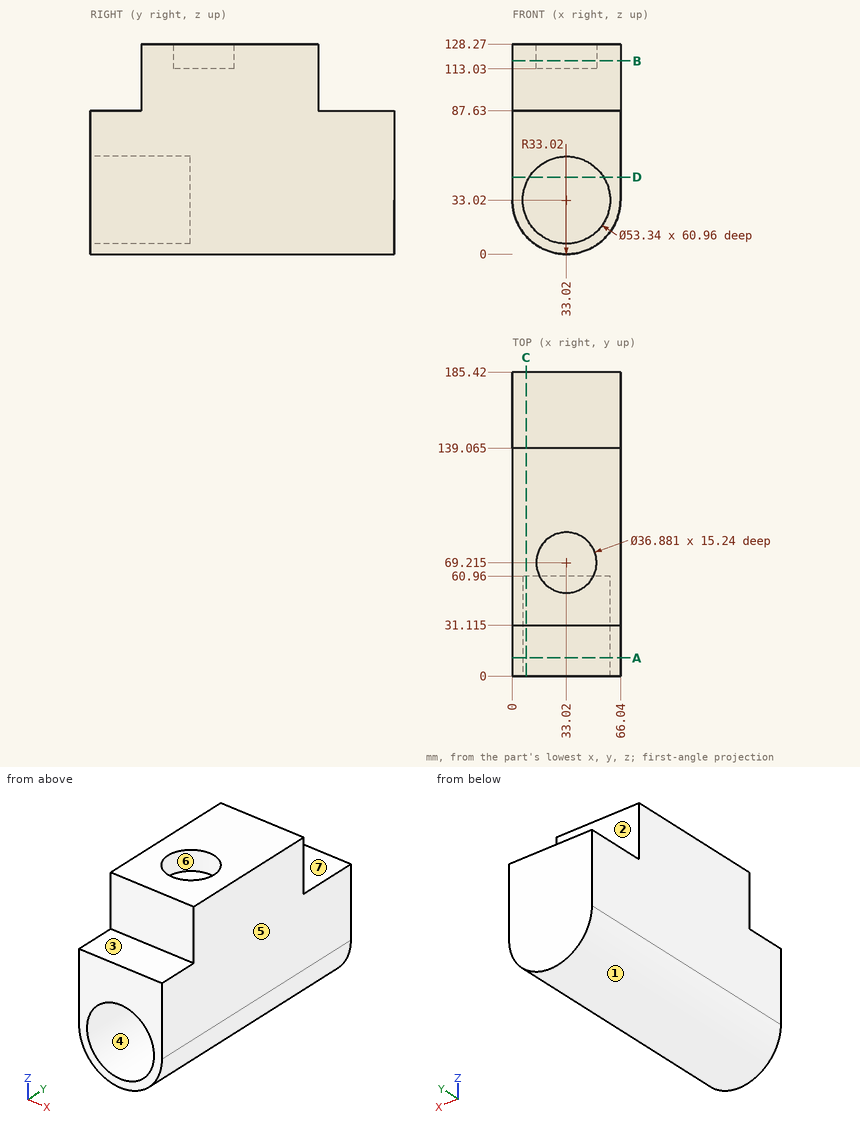
Here's the drawing with two shaded views (mm, measured from the low corner). I have some questions. A direction names the side the tool comes from. Give positions to 0.01 mm unless a question says otherwise; leave off trailing zeros. Loops run counter-clockwise (first coordinate to the right, second up) from the corner with the lowest first, then second, coordinate; pieces in that order, holes last. Notation, with made-up numbers: M 15,52.5 L 61,52.5 A25 ccw 61,86.5 Z; hole C 73,63 d10. An arc over 180 degrees is marked long. One line per item, written item: value.
(1) We'd pull the mould along X, two halves only. Please class the marked faces 4, 5, 6 and 7: released by +X, released by -X, zero draft, split by the parting line, or undercut.
Returned:
face 4: undercut
face 5: released by +X
face 6: undercut
face 7: zero draft
(2) Will these pins go through, and if not, where does the flat tip stop? pin 1 (12 mm diameter, centred on x = 28.5, z = 112.5, fed in from -Y) (3 decimals); pin 2 (16 mm diameter, centred on x = 42.5, z = 41, fed in from -Y); pin 3 (15.5 mm diameter, centred on x = 41.5, y = 22.5, fed in from +Z).
Returned:
pin 1: y = 31.115
pin 2: y = 60.96
pin 3: z = 87.63
(3) Suppose I cut it at B-B on z = 118. List the corners of the cut face in (x, y) for me (1 decimal).
Returned:
outline: M 0,31.1 L 66,31.1 L 66,139.1 L 0,139.1 Z; hole C 33,69.2 d36.9
(4) Suppose I cut it at C-C on x = 8.5. List the corners of the cut face in (y, z) for me (1 decimal).
Returned:
outline: M 0,10.9 L 185.4,10.9 L 185.4,87.6 L 139.1,87.6 L 139.1,128.3 L 31.1,128.3 L 31.1,87.6 L 0,87.6 L 0,43.5 L 61,43.5 L 61,22.5 L 0,22.5 Z
(5) Suppose I cut it at A-A on y = 11. List the corners of the cut face in (x, z) for me, plus the area to 3 significant figures.
Returned:
outline: M 0,33.02 A33.02 ccw 66.04,33.02 L 66.04,87.63 L 0,87.63 Z; hole C 33.02,33.02 d53.34
area: 3,080 mm^2
(6) Suppose I cut it at D-D on z = 47. List the corners of the cut face in (x, y) for me.
Returned:
outline: M 0,0 L 10.31,0 L 10.31,60.96 L 55.73,60.96 L 55.73,0 L 66.04,0 L 66.04,185.42 L 0,185.42 Z
(7) I need wall thicknesses on line 1 (Z direction, x = 33, y = 44); line 2 (Y direction, x = 33.02, z = 120) (1 decimal); line 3 (Z direction, x = 34, y = 57.5). Which ranges of each line are inside material? Lowest first, please.
Returned:
line 1: 0 to 6.35, 59.69 to 128.27
line 2: 31.1 to 50.8, 87.7 to 139.1
line 3: 0.01 to 6.37, 59.67 to 113.03
(8) Which directions (+Z, -Z, +X, -X, +Y, -Y) give clear straight access to the entire face, cutting with the end or side of a thin tool? Please do the marked faces 1, 2 and 3.
Returned:
face 1: -Z, +Y, -Y
face 2: +Z, +X, -X, +Y
face 3: +Z, +X, -X, -Y
